Autodesk Inventor part; units mm, degrees
ref_plane "YZ Plane" through (0, 0, 0) normal (1, 0, 0) x (0, 1, 0)
ref_plane "XZ Plane" through (0, 0, 0) normal (0, 1, 0) x (-1, 0, 0)
ref_plane "XY Plane" through (0, 0, 0) normal (0, 0, 1) x (1, 0, 0)
sketch "Sketch1" plane through (0, 0, 0) normal (0, 0, 1) x (1, 0, 0)
  circle A0 centre (0, 0) radius 7.62
  line L0 (-10.16, 7.62) -> (-10.16, 0)
  arc A1 (-10.16, 0) -> (10.16, 0) centre (0, 0) ccw
  line L1 (10.16, 0) -> (10.16, 7.62)
  line L2 (10.16, 7.62) -> (7.62, 7.62)
  line L3 (7.62, 7.62) -> (7.62, 0)
  line L4 (-10.16, 7.62) -> (-7.62, 7.62)
  line L5 (-7.62, 7.62) -> (-7.62, 0)
  dimension "d0" = 15.24
  dimension "d1" = 2.54
  dimension "d2" = 2.54
  dimension "d3" = 2.54
extrude "Extrusion1" add sketch "Sketch1" along normal blind 152.4 contours L3 L2 L1 A1 L0 L4 L5 A0
sketch "Sketch2" plane through (-7.62, 0, 0) normal (1, 0, 0) x (0, 0, -1)
  line L0 (0, 7.62) -> (-152.4, 7.62)
  line L1 (0, 7.62) -> (-6.35, 7.62)
  line L2 (-6.35, 7.62) -> (-6.35, 13.97)
  line L3 (-6.35, 13.97) -> (0, 13.97)
  line L4 (0, 13.97) -> (0, 7.62)
  circle A0 centre (-3.175, 10.795) radius 1.27
  point P0 (0, 0)
  dimension "d6" = 6.35
  dimension "d7" = 6.35
  dimension "d8" = 2.54
  dimension "d9" = 3.175
  dimension "d10" = 3.175
extrude "Extrusion2" add sketch "Sketch2" against normal up to surface (2.54 mm away)
sketch "Sketch4" plane through (-7.62, 0, 152.4) normal (1, 0, 0) x (0, 0, -1)
  line L0 (0, 0) -> (0, 7.62)
  circle A0 centre (3.175, 10.473) radius 1.27
  line L1 (152.4, 7.62) -> (0, 7.62)
  line L2 (6.35, 7.62) -> (0, 7.62)
  line L3 (0, 7.62) -> (6.35, 7.62)
  line L4 (6.35, 7.62) -> (6.35, 13.97)
  line L5 (6.35, 13.97) -> (0, 13.97)
  line L6 (0, 13.97) -> (0, 7.62)
  point P0 (152.4, 0)
  dimension "d15" = 2.54
  dimension "d16" = 6.35
  dimension "d17" = 6.35
extrude "Extrusion3" add sketch "Sketch4" against normal up to surface (2.54 mm away)
properties part number "StraightTrack"
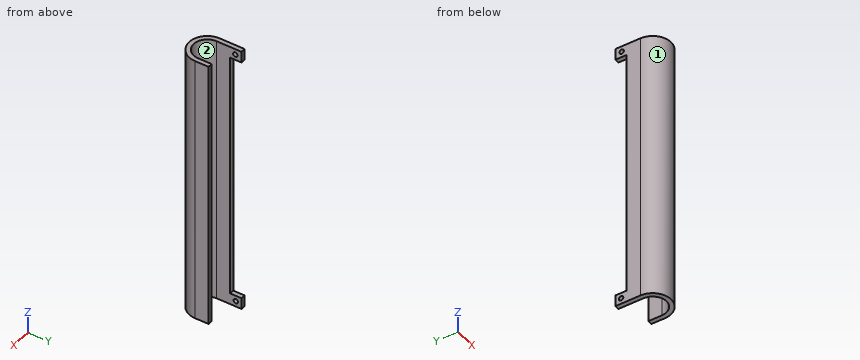
The model under review builds one solid part; all positions refer to its coordinate system, in mm. Face numbers are marked on the shaded views. Give positions to 0.01 mm unless a question says otherwise; leave off trailing zeros. Order: outer loops, then holes, each group sorted by start corner. A loop starts at its lowest first (then second) coordinate and runs counter-clockwise, first axis right, second up. Notation, with made-up numbers: M 82.25,-19.5 L 125.25,-19.5 A21 ccw 125.25,-6.5 Z; hole C -39.75,46.5 d4. An arc over 180 degrees is marked long. Use one line per item in the form item = value. Start each with the question number.
Item 1: We need section B-B on z = 50. Give the boundary of the cut face in (x, y), plus the area to 3 significant figures.
Item 2: The part is to be moulded in two halves that separate along X. For the marked faces 1 and 2, say which applies: pulls with the +X half, pulls with the -X half, needs draft (parallel to the pull), parting line crosses it, or undercut.
Item 3: Insertion check: pin 1 Ø1.5 at (x, z) = (-5.5, 90.5) entering from +Y; pin 2 Ø3 at (y, z) = (-7, 30) entering from +X; pin 3 Ø1 at (x, z) = (-4.5, 29) entering from +Y. Each pin has a flat end and moves straight along its axis. Give the tip position at first contact, or say it passes through.
Item 4: We need section A-A on y = 4.5. Give the boundary of the cut face in (x, z).
Item 5: We need section D-D on y = -1.75. Give the boundary of the cut face in (x, z), plus the area to 3 significant figures.
Item 6: We need section C-C on x = 0. Give the boundary of the cut face in (y, z).
Item 7: To check wall thickness, follow line 1 along X through (y, z) = (1.25, 119); line 2 along X through (y, z) = (-1, 29); line 3 along Y through (x, z) = (0, 94.5). State the ranges of each line that lie inside material, in increasing order. Write a range as from..to.
Completed:
q1.outline = M -10.16,0 A10.16 ccw 10.16,0 L 10.16,7.62 L 7.62,7.62 L 7.62,0 A7.62 cw -7.62,0 L -7.62,7.62 L -10.16,7.62 Z
q1.area = 110 mm²
q2.face_1 = parting line crosses it
q2.face_2 = undercut
q3.pin_1 = -4.36
q3.pin_2 = 8.54
q3.pin_3 = -5.75
q4.outline = M -10.16,0 L -7.62,0 L -7.62,152.4 L -10.16,152.4 Z; M 7.62,0 L 10.16,0 L 10.16,152.4 L 7.62,152.4 Z
q5.outline = M -10.01,0 L -7.42,0 L -7.42,152.4 L -10.01,152.4 Z; M 7.42,0 L 10.01,0 L 10.01,152.4 L 7.42,152.4 Z
q5.area = 790 mm²
q6.outline = M -10.16,0 L -7.62,0 L -7.62,152.4 L -10.16,152.4 Z
q7.line_1 = -10.16..-7.62, 7.62..10.16
q7.line_2 = -10.11..-7.55, 7.55..10.11
q7.line_3 = -10.16..-7.62
